Can you work these out from the model? Positions are in its coordinate system, mm. Coordinates: 2 decimals unless noted, no trailing zeros. Order: outer loops, then holes, each group sorted by start corner. A loop starts at its lowest first (then second) coordinate and runs counter-clockwise, first axis right, second up. Notation, with made-up numbers: M 0,32.25 L 58,32.25 A26 ccw 58,65.25 Z; hole C -27,-4.5 d2. An arc over 180 degrees is marked long. Answer as a JSON object with one key per item and string values.
from build123d import *

# Parameters (mm, degrees)
SKETCH_1_W               = 96
SKETCH_1_H               = 96
EXTRUDE_1_DEPTH          = 3
CUT_EXTRUDE_1_REACH      = 69.949
SKETCH_3_R               = 2.75
MIRROR_2_COPY_1_REACH    = 69.949
MIRROR_2_COPY_1_SKETCH_R = 2.75


with BuildPart() as part:
    # Sketch 1 → Extrude 1 (new body)
    with BuildSketch(Plane(origin=(0, 0, 0), x_dir=(1, 0, 0), z_dir=(0, 1, 0))):
        Rectangle(SKETCH_1_W, SKETCH_1_H)
    extrude(amount=EXTRUDE_1_DEPTH)

    # Sketch 3 → Cut-Extrude 1 (cut, up to next)
    with BuildSketch(Plane(origin=(0, 3, 0), x_dir=(1, 0, 0), z_dir=(0, 1, 0)), mode=Mode.PRIVATE) as cut_extrude_1_sk1:
        with Locations(Location((-14, 14, 0), (0, 0, 270))):
            Circle(SKETCH_3_R)
    cut_extrude_1_tool1 = extrude(cut_extrude_1_sk1.sketch, amount=-CUT_EXTRUDE_1_REACH, mode=Mode.PRIVATE) & part.part
    # Sketch 3 → Cut-Extrude 1 (cut, up to next)
    with BuildSketch(Plane(origin=(0, 3, 0), x_dir=(1, 0, 0), z_dir=(0, 1, 0)), mode=Mode.PRIVATE) as cut_extrude_1_sk2:
        Polygon((-27.75, 35.25), (-19, 35.25), (-19, 27.75), (-27.75, 27.75), (-27.75, 19), (-35.25, 19), (-35.25, 27.75), (-44, 27.75), (-44, 35.25), (-35.25, 35.25), (-35.25, 44), (-27.75, 44), align=None)
    cut_extrude_1_tool2 = extrude(cut_extrude_1_sk2.sketch, amount=-CUT_EXTRUDE_1_REACH, mode=Mode.PRIVATE) & part.part
    # Sketch 3 → Cut-Extrude 1 (cut, up to next)
    with BuildSketch(Plane(origin=(0, 3, 0), x_dir=(1, 0, 0), z_dir=(0, 1, 0)), mode=Mode.PRIVATE) as cut_extrude_1_sk3:
        Polygon((-41, 44), (-39, 44), (-39, 39), (-43, 39), (-43, 41), (-41, 41), align=None)
    cut_extrude_1_tool3 = extrude(cut_extrude_1_sk3.sketch, amount=-CUT_EXTRUDE_1_REACH, mode=Mode.PRIVATE) & part.part
    # Sketch 3 → Cut-Extrude 1 (cut, up to next)
    with BuildSketch(Plane(origin=(0, 3, 0), x_dir=(1, 0, 0), z_dir=(0, 1, 0)), mode=Mode.PRIVATE) as cut_extrude_1_sk4:
        Polygon((-22, 41), (-22, 44), (-24, 44), (-24, 39), (-20, 39), (-20, 41), align=None)
    cut_extrude_1_tool4 = extrude(cut_extrude_1_sk4.sketch, amount=-CUT_EXTRUDE_1_REACH, mode=Mode.PRIVATE) & part.part
    # Sketch 3 → Cut-Extrude 1 (cut, up to next)
    with BuildSketch(Plane(origin=(0, 3, 0), x_dir=(1, 0, 0), z_dir=(0, 1, 0)), mode=Mode.PRIVATE) as cut_extrude_1_sk5:
        Polygon((-22, 19), (-24, 19), (-24, 24), (-20, 24), (-20, 22), (-22, 22), align=None)
    cut_extrude_1_tool5 = extrude(cut_extrude_1_sk5.sketch, amount=-CUT_EXTRUDE_1_REACH, mode=Mode.PRIVATE) & part.part
    # Sketch 3 → Cut-Extrude 1 (cut, up to next)
    with BuildSketch(Plane(origin=(0, 3, 0), x_dir=(1, 0, 0), z_dir=(0, 1, 0)), mode=Mode.PRIVATE) as cut_extrude_1_sk6:
        Polygon((-41, 22), (-41, 19), (-39, 19), (-39, 24), (-43, 24), (-43, 22), align=None)
    cut_extrude_1_tool6 = extrude(cut_extrude_1_sk6.sketch, amount=-CUT_EXTRUDE_1_REACH, mode=Mode.PRIVATE) & part.part
    cut_extrude_1_1 = cut_extrude_1_tool1.solids().sort_by_distance((-14, 3, -14))[0]
    add(cut_extrude_1_1, mode=Mode.SUBTRACT)
    cut_extrude_1_2 = cut_extrude_1_tool2.solids().sort_by_distance((-31.5, 3, -31.5))[0]
    add(cut_extrude_1_2, mode=Mode.SUBTRACT)
    cut_extrude_1_3 = cut_extrude_1_tool3.solids().sort_by_distance((-40.571429, 3, -41.071429))[0]
    add(cut_extrude_1_3, mode=Mode.SUBTRACT)
    cut_extrude_1_4 = cut_extrude_1_tool4.solids().sort_by_distance((-22.428571, 3, -41.071429))[0]
    add(cut_extrude_1_4, mode=Mode.SUBTRACT)
    cut_extrude_1_5 = cut_extrude_1_tool5.solids().sort_by_distance((-22.428571, 3, -21.928571))[0]
    add(cut_extrude_1_5, mode=Mode.SUBTRACT)
    cut_extrude_1_6 = cut_extrude_1_tool6.solids().sort_by_distance((-40.571429, 3, -21.928571))[0]
    add(cut_extrude_1_6, mode=Mode.SUBTRACT)
    cut_extrude_1 = cut_extrude_1_1 + cut_extrude_1_2 + cut_extrude_1_3 + cut_extrude_1_4 + cut_extrude_1_5 + cut_extrude_1_6  # Cut-Extrude 1 as one shape, for the pattern or mirror that repeats it

    # Mirror 1: Cut-Extrude 1 across plane
    add(cut_extrude_1.mirror(Plane(origin=(0, 0, 0), x_dir=(0, 0, 1), z_dir=(1, 0, 0))), mode=Mode.SUBTRACT)

    # Mirror 2: Cut-Extrude 1 across plane
    add(cut_extrude_1.mirror(Plane.XY), mode=Mode.SUBTRACT)

    # Mirror 2 copy 1 sketch → Mirror 2 copy 1 (cut, up to next)
    with BuildSketch(Plane(origin=(0, 3, 0), x_dir=(-1, 0, 0), z_dir=(0, 1, 0)), mode=Mode.PRIVATE) as mirror_2_copy_1_sk1:
        with Locations(Location((-14, 14, 0), (0, 0, 270))):
            Circle(MIRROR_2_COPY_1_SKETCH_R)
    mirror_2_copy_1_tool1 = extrude(mirror_2_copy_1_sk1.sketch, amount=-MIRROR_2_COPY_1_REACH, mode=Mode.PRIVATE) & part.part
    # Mirror 2 copy 1 sketch → Mirror 2 copy 1 (cut, up to next)
    with BuildSketch(Plane(origin=(0, 3, 0), x_dir=(-1, 0, 0), z_dir=(0, 1, 0)), mode=Mode.PRIVATE) as mirror_2_copy_1_sk2:
        Polygon((-27.75, 35.25), (-19, 35.25), (-19, 27.75), (-27.75, 27.75), (-27.75, 19), (-35.25, 19), (-35.25, 27.75), (-44, 27.75), (-44, 35.25), (-35.25, 35.25), (-35.25, 44), (-27.75, 44), align=None)
    mirror_2_copy_1_tool2 = extrude(mirror_2_copy_1_sk2.sketch, amount=-MIRROR_2_COPY_1_REACH, mode=Mode.PRIVATE) & part.part
    # Mirror 2 copy 1 sketch → Mirror 2 copy 1 (cut, up to next)
    with BuildSketch(Plane(origin=(0, 3, 0), x_dir=(-1, 0, 0), z_dir=(0, 1, 0)), mode=Mode.PRIVATE) as mirror_2_copy_1_sk3:
        Polygon((-41, 44), (-39, 44), (-39, 39), (-43, 39), (-43, 41), (-41, 41), align=None)
    mirror_2_copy_1_tool3 = extrude(mirror_2_copy_1_sk3.sketch, amount=-MIRROR_2_COPY_1_REACH, mode=Mode.PRIVATE) & part.part
    # Mirror 2 copy 1 sketch → Mirror 2 copy 1 (cut, up to next)
    with BuildSketch(Plane(origin=(0, 3, 0), x_dir=(-1, 0, 0), z_dir=(0, 1, 0)), mode=Mode.PRIVATE) as mirror_2_copy_1_sk4:
        Polygon((-22, 41), (-22, 44), (-24, 44), (-24, 39), (-20, 39), (-20, 41), align=None)
    mirror_2_copy_1_tool4 = extrude(mirror_2_copy_1_sk4.sketch, amount=-MIRROR_2_COPY_1_REACH, mode=Mode.PRIVATE) & part.part
    # Mirror 2 copy 1 sketch → Mirror 2 copy 1 (cut, up to next)
    with BuildSketch(Plane(origin=(0, 3, 0), x_dir=(-1, 0, 0), z_dir=(0, 1, 0)), mode=Mode.PRIVATE) as mirror_2_copy_1_sk5:
        Polygon((-22, 19), (-24, 19), (-24, 24), (-20, 24), (-20, 22), (-22, 22), align=None)
    mirror_2_copy_1_tool5 = extrude(mirror_2_copy_1_sk5.sketch, amount=-MIRROR_2_COPY_1_REACH, mode=Mode.PRIVATE) & part.part
    # Mirror 2 copy 1 sketch → Mirror 2 copy 1 (cut, up to next)
    with BuildSketch(Plane(origin=(0, 3, 0), x_dir=(-1, 0, 0), z_dir=(0, 1, 0)), mode=Mode.PRIVATE) as mirror_2_copy_1_sk6:
        Polygon((-41, 22), (-41, 19), (-39, 19), (-39, 24), (-43, 24), (-43, 22), align=None)
    mirror_2_copy_1_tool6 = extrude(mirror_2_copy_1_sk6.sketch, amount=-MIRROR_2_COPY_1_REACH, mode=Mode.PRIVATE) & part.part
    add(mirror_2_copy_1_tool1.solids().sort_by_distance((14, 3, 14))[0], mode=Mode.SUBTRACT)
    add(mirror_2_copy_1_tool2.solids().sort_by_distance((31.5, 3, 31.5))[0], mode=Mode.SUBTRACT)
    add(mirror_2_copy_1_tool3.solids().sort_by_distance((40.571429, 3, 41.071429))[0], mode=Mode.SUBTRACT)
    add(mirror_2_copy_1_tool4.solids().sort_by_distance((22.428571, 3, 41.071429))[0], mode=Mode.SUBTRACT)
    add(mirror_2_copy_1_tool5.solids().sort_by_distance((22.428571, 3, 21.928571))[0], mode=Mode.SUBTRACT)
    add(mirror_2_copy_1_tool6.solids().sort_by_distance((40.571429, 3, 21.928571))[0], mode=Mode.SUBTRACT)


solid = part.part
Item 1: I want a section at C-C, the plane y = 1.05. Give the number of separate pieces and of enclosed holes in the cut face, plus the area to 3 significant figures.
Answers follow:
{"separate pieces": "1", "enclosed holes": "24", "area": "7,620 mm^2"}
Item 2: I want a section at B-B, the plane x = -14. Write out the boundary of the cut face in (y, z).
Answers follow:
{"outline": "M 0,-48 L 3,-48 L 3,-16.75 L 0,-16.75 Z; M 0,-11.25 L 3,-11.25 L 3,11.25 L 0,11.25 Z; M 0,16.75 L 3,16.75 L 3,48 L 0,48 Z"}
Item 3: I want a section at A-A, the plane z = -14. Write out the boundary of the cut face in (x, y).
Answers follow:
{"outline": "M -48,0 L -16.75,0 L -16.75,3 L -48,3 Z; M -11.25,0 L 11.25,0 L 11.25,3 L -11.25,3 Z; M 16.75,0 L 48,0 L 48,3 L 16.75,3 Z"}
Item 4: Please list where these lines run through material, in increasing order: line 1 (X direction, y = 1, z = -14); line 2 (Z direction, x = -30, y = 2.5).
Answers follow:
{"line 1": "x = -48 to -16.75, -11.25 to 11.25, 16.75 to 48", "line 2": "z = -48 to -44, -19 to 19, 44 to 48"}
Item 5: If we mould it in two halves opening along X, with no side actions, what happens to faces 1 (the flat face through (22, 2, 42)), 2 (the flat face through (32, 2, 44))? For each: pulls with the +X half, pulls with the -X half, needs draft (parallel to the pull), parting line crosses it, or undercut.
Answers follow:
{"face 1": "undercut", "face 2": "undercut"}
